Here's how the part is built. I have some questions about the finished solid (model axes, mm). Round coordinates to 2 decimals unless told otherwise and drop trailing zeros. Loops run counter-clockwise (first coordinate to the right, second up) from the corner with the lowest first, then second, coordinate; pieces in that order, holes last. Notation, with made-up numbers: M 30,-11 L 81,-11 A19 ccw 81,15 Z; hole C 30,-10.5 d8. An arc over 180 degrees is marked long. Answer as a JSON object with one key per item and string values.
from build123d import *

# Parameters (mm, degrees)
EXTRUDE_1_DEPTH        = 10
SKETCH_3_W             = 140
SKETCH_3_H             = 3
CUT_EXTRUDE_1_DEPTH    = 10
CUT_EXTRUDE_2_DEPTH    = 10
HOLE_WIZARD_M5_3_D     = 4.2
HOLE_WIZARD_M5_3_DEPTH = 14
HOLE_WIZARD_M5_3_TIP   = 1.2618073
HOLE_WIZARD_M6_2_D     = 5
HOLE_WIZARD_M6_2_DEPTH = 17
HOLE_WIZARD_M6_2_TIP   = 1.502151548
SKETCH_10_W            = 15
SKETCH_10_H            = 2.5
CUT_EXTRUDE_3_DEPTH    = 7
SKETCH_11_R            = 1.5
CUT_EXTRUDE_4_DEPTH    = 11
SKETCH_13_R            = 2
CUT_EXTRUDE_6_DEPTH    = 5
SKETCH_14_R            = 2
CUT_EXTRUDE_7_DEPTH    = 5
SKETCH_16_R            = 1.5
CUT_EXTRUDE_8_DEPTH    = 10


with BuildPart() as part:
    # 草图1 → 凸台-拉伸1 (new body)
    with BuildSketch(Plane.XY):
        with BuildLine():
            Line((-197, 12.5), (197, 12.5))
            ThreePointArc((197, 12.5), (199.121320344, 11.621320344), (200, 9.5))
            Line((200, 9.5), (200, -9.5))
            ThreePointArc((200, -9.5), (199.121320344, -11.621320344), (197, -12.5))
            Line((197, -12.5), (-197, -12.5))
            ThreePointArc((-197, -12.5), (-199.121320344, -11.621320344), (-200, -9.5))
            Line((-200, -9.5), (-200, 9.5))
            ThreePointArc((-200, 9.5), (-199.121320344, 11.621320344), (-197, 12.5))
        make_face()
    extrude(amount=-EXTRUDE_1_DEPTH)

    # 草图3 → 切除-拉伸1 (cut)
    with BuildSketch(Plane.XY):
        with Locations((0, 9)):
            Rectangle(SKETCH_3_W, SKETCH_3_H)
    extrude(amount=-CUT_EXTRUDE_1_DEPTH, mode=Mode.SUBTRACT)

    # 草图4 → 切除-拉伸2 (cut)
    with BuildSketch(Plane.XY):
        with BuildLine():
            ThreePointArc((-190, 10.5), (-191.414213562, 9.914213562), (-192, 8.5))
            Line((-192, 8.5), (-190, 8.5))
            Line((-190, 8.5), (-190, 10.5))
        make_face()
        with BuildLine():
            Line((-190, 8.5), (-192, 8.5))
            ThreePointArc((-192, 8.5), (-191.414213562, 7.085786438), (-190, 6.5))
            Line((-190, 6.5), (-190, 8.5))
        make_face()
        with BuildLine():
            Line((-190, 10.5), (-190, 8.5))
            Line((-190, 8.5), (-188, 8.5))
            ThreePointArc((-188, 8.5), (-188.585786438, 9.914213562), (-190, 10.5))
        make_face()
        with BuildLine():
            Line((-188, 8.5), (-190, 8.5))
            Line((-190, 8.5), (-190, 6.5))
            ThreePointArc((-190, 6.5), (-188.585786438, 7.085786438), (-188, 8.5))
        make_face()
        with BuildLine():
            ThreePointArc((190, 10.5), (188.585786438, 9.914213562), (188, 8.5))
            Line((188, 8.5), (190, 8.5))
            Line((190, 8.5), (190, 10.5))
        make_face()
        with BuildLine():
            Line((190, 8.5), (188, 8.5))
            ThreePointArc((188, 8.5), (188.585786438, 7.085786438), (190, 6.5))
            Line((190, 6.5), (190, 8.5))
        make_face()
        with BuildLine():
            Line((190, 10.5), (190, 8.5))
            Line((190, 8.5), (192, 8.5))
            ThreePointArc((192, 8.5), (191.414213562, 9.914213562), (190, 10.5))
        make_face()
        with BuildLine():
            Line((192, 8.5), (190, 8.5))
            Line((190, 8.5), (190, 6.5))
            ThreePointArc((190, 6.5), (191.414213562, 7.085786438), (192, 8.5))
        make_face()
    extrude(amount=-CUT_EXTRUDE_2_DEPTH, mode=Mode.SUBTRACT)

    # M5 螺纹孔3
    with Locations(Plane.XY):
        with Locations((-150, 0), (-83, 0), (-36, 0)):
            Hole(HOLE_WIZARD_M5_3_D / 2, depth=HOLE_WIZARD_M5_3_DEPTH)
            with Locations((0, 0, -(HOLE_WIZARD_M5_3_DEPTH + HOLE_WIZARD_M5_3_TIP / 2))):  # 118° drill point
                Cone(0, HOLE_WIZARD_M5_3_D / 2, HOLE_WIZARD_M5_3_TIP, mode=Mode.SUBTRACT)

    # M6 螺纹孔2
    with Locations(Plane.XY):
        with Locations((-46, 0), (-136, 0)):
            Hole(HOLE_WIZARD_M6_2_D / 2, depth=HOLE_WIZARD_M6_2_DEPTH)
            with Locations((0, 0, -(HOLE_WIZARD_M6_2_DEPTH + HOLE_WIZARD_M6_2_TIP / 2))):  # 118° drill point
                Cone(0, HOLE_WIZARD_M6_2_D / 2, HOLE_WIZARD_M6_2_TIP, mode=Mode.SUBTRACT)

    # 草图10 → 切除-拉伸3 (cut)
    with BuildSketch(Plane.XZ.offset(12.5)):
        with Locations((-172.5, -3.75)):
            Rectangle(SKETCH_10_W, SKETCH_10_H)
        with Locations((-157.5, -3.75)):
            Rectangle(SKETCH_10_W, SKETCH_10_H)
        with Locations((-157.5, -6.25)):
            Rectangle(SKETCH_10_W, SKETCH_10_H)
        with Locations((-172.5, -6.25)):
            Rectangle(SKETCH_10_W, SKETCH_10_H)
        with Locations((157.5, -3.75)):
            Rectangle(SKETCH_10_W, SKETCH_10_H)
        with Locations((172.5, -3.75)):
            Rectangle(SKETCH_10_W, SKETCH_10_H)
        with Locations((157.5, -6.25)):
            Rectangle(SKETCH_10_W, SKETCH_10_H)
        with Locations((172.5, -6.25)):
            Rectangle(SKETCH_10_W, SKETCH_10_H)
    extrude(amount=-CUT_EXTRUDE_3_DEPTH, mode=Mode.SUBTRACT)

    # 草图11 → 切除-拉伸4 (cut, through all)
    with BuildSketch(Plane.XY):
        with Locations((-165, -9)):
            Circle(SKETCH_11_R)
        with Locations((165.001644556, -9)):
            Circle(SKETCH_11_R)
    extrude(amount=-CUT_EXTRUDE_4_DEPTH, mode=Mode.SUBTRACT)

    # 草图13 → 切除-拉伸6 (cut)
    with BuildSketch(Plane(origin=(200, 0, 0), x_dir=(0, 0, -1), z_dir=(1, 0, 0))):
        with Locations((5, 0)):
            Circle(SKETCH_13_R)
    extrude(amount=-CUT_EXTRUDE_6_DEPTH, mode=Mode.SUBTRACT)

    # 草图14 → 切除-拉伸7 (cut)
    with BuildSketch(Plane.ZY.offset(200)):
        with Locations((-5, 0)):
            Circle(SKETCH_14_R)
    extrude(amount=-CUT_EXTRUDE_7_DEPTH, mode=Mode.SUBTRACT)

    # 草图16 → 切除-拉伸8 (cut)
    with BuildSketch(Plane(origin=(0, 12.5, 0), x_dir=(1, 0, 0), z_dir=(0, 1, 0))):
        with Locations((0, 5)):
            Circle(SKETCH_16_R)
    extrude(amount=-CUT_EXTRUDE_8_DEPTH, mode=Mode.SUBTRACT)


solid = part.part
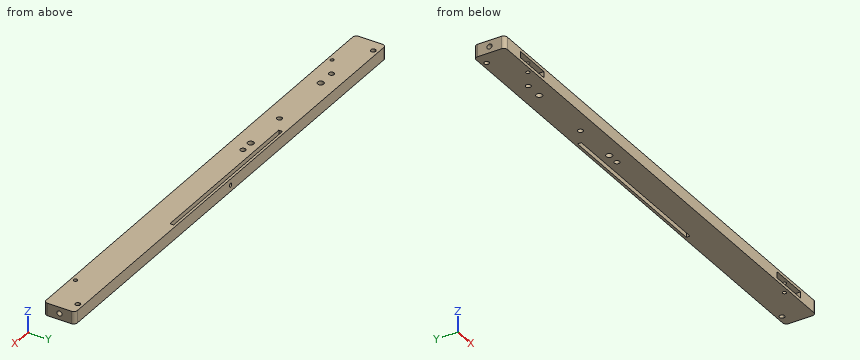
Item 1: I want a section at B-B, the plane z = -5. State how many separate pieces and enclosed holes the cut face has, then the cut area to 3 significant figures.
Resolved:
{"separate pieces": "1", "enclosed holes": "7", "area": "8,990 mm²"}
Item 2: I want a section at A-A, the plane x = -30.5. Please give me the cut outline in (y, z).
Resolved:
{"outline": "M -12.5,-10 L 7.5,-10 L 7.5,0 L -12.5,0 Z; M 10.5,-10 L 12.5,-10 L 12.5,0 L 10.5,0 Z"}
Item 3: Please list where these lines run through material, in increasing order: probe 1 along X at (y, z) = (-6.75, -6.75); probe 2 along X at (y, z) = (0.5, -6); probe 3 along X at (y, z) = (8, -7). Write a range as from..to.
Resolved:
{"probe 1": "-200..-180, -150..150, 180..200", "probe 2": "-195..-152.04, -147.96..-138.45, -133.55..-85.04, -80.96..-48.45, -43.55..-38.04, -33.96..195", "probe 3": "-200..-191.94, -188.06..-70, 70..188.06, 191.94..200"}
Item 4: I'm going to push a flat-ended pin straight in: pin 1 Ø1.2 at (y, z) = (0.5, -5.5) entering from -X. Where does the tip first touch, or does it pass through?
Resolved:
{"pin 1": "x = -195"}
